Build history of the part. All positions in model axes, mm. Face numbers are marked on the shaded views. A direction names the side the tool comes from. Round coordinates to 2 decimals unless told otherwise and drop trailing zeros. Order: outer loops, then holes, each group sorted by start corner. A loop starts at its lowest first (then second) coordinate and runs counter-clockwise, first axis right, second up. Notation, with made-up numbers: M 8.5,-0.5 L 39.5,-0.5 A21 cw 39.5,7.5 Z; hole C 12.5,46 d6. An arc over 180 degrees is marked long. One line per item, written item: value. Start each with the question number.
Item 1: Two-plate mould, pull along Y, no slides. Class the marked faces 3, 4, 5 and 6: +Y half, -Y half, draft (parallel to the pull), parting line (faces both ways), or undercut.
Item 2: Band-saw the part on A-A, the plane x = 0. Write the cut outline in (y, z).
Item 3: Band-saw the part on C-C, the plane y = -4. Write the cut outline in (x, z), then the cut area to 3 significant figures.
Item 4: Probe L1, parallel to Y at x = 0, z = 0.4; L2, parallel to X at y = -4, z = 0.7; L3, parallel to Z at x = -2, y = -5.25. List the from-to ranges inside material, lowest first.
Item 5: Band-saw the part on D-D, the plane z = 1.75. Write the cut outline in (x, y).
Item 6: Pin check, flat tips, straight feed: pin 1 (4 mm diameter, centred on x = 6.5, y = -4, fed in from +Z); pin 2 (4 mm diameter, centred on x = 2, z = 6.5, fed in from -Y); pin 3 (2 mm diameter, centred on x = 0.5, y = -6, fed in from +Z). Stop position of each tip, or through.
Item 7: Tool access for the marked faces 1 and 2: list every direction of +Z, -Z, +X, -X, +Y, -Y with a clear straight run to the whole face (end or side of a thin tool).
Item 8: Band-saw the part on B-B, the plane y = 8. Write the cut outline in (x, z).
```python
from build123d import *

# Parameters (mm, degrees)
SKETCH_1_R               = 3
SKETCH_1_R_2             = 1.65
EXTRUDE_1_DEPTH          = 4
CUT_EXTRUDE_2_DEPTH      = 6.830951895
PATTERN_CIRCULAR_1_COUNT = 9
SKETCH_2_R               = 5
EXTRUDE_2_DEPTH          = 4
SKETCH_3_R               = 12.5
SKETCH_3_R_2             = 1.8
SKETCH_3_R_3             = 5
EXTRUDE_4_DEPTH          = 4
CUT_EXTRUDE_START        = 4
SKETCH_3_3_R             = 2.5
CUT_EXTRUDE_3_DEPTH      = 3
SKETCH_4_R               = 1.4
EXTRUDE_5_DEPTH          = 12.5


with BuildPart() as part:
    # 草图1 → 凸台-拉伸1 (new body)
    with BuildSketch(Plane.XY):
        Circle(SKETCH_1_R)
        Circle(SKETCH_1_R_2, mode=Mode.SUBTRACT)
    extrude(amount=EXTRUDE_1_DEPTH)

    # 草图1<3> → 切除-拉伸2 (cut, through all)
    with BuildSketch(Plane.XY):
        with BuildLine():
            Line((1.583201231, 0.595370355), (1.54440693, 0.580781573))
            ThreePointArc((1.54440693, 0.580781573), (1.623387112, 0.295151288), (1.65, 0))
            ThreePointArc((1.65, 0), (1.623387112, -0.295151288), (1.54440693, -0.580781573))
            Line((1.54440693, -0.580781573), (1.583201231, -0.595370355))
            add(Edge.make_bspline(
                [(1.583201231, -0.595370355), (1.595268082, -0.599908151), (1.629927649, -0.609960022), (1.698544644, -0.618780808), (1.810680065, -0.617601716), (1.954246735, -0.59352555), (2.132298369, -0.536822163), (2.302941373, -0.452472776), (2.42578745, -0.372108406), (2.505673341, -0.310927028), (2.533645284, -0.288342805)],
                knots=[0, 0, 0, 0, 0, 0.005604068, 0.015718248, 0.029959916, 0.048733667, 0.068727063, 0.096888892, 0.112551479, 0.112551479, 0.112551479, 0.112551479, 0.112551479], degree=4))
            ThreePointArc((2.533645284, -0.288342805), (2.545908038, -0.144403125), (2.55, 0))
            ThreePointArc((2.55, 0), (2.545908038, 0.144403125), (2.533645284, 0.288342805))
            add(Edge.make_bspline(
                [(1.583201231, 0.595370355), (1.595268082, 0.599908151), (1.629927649, 0.609960022), (1.698544644, 0.618780808), (1.810680065, 0.617601716), (1.954246735, 0.59352555), (2.132298369, 0.536822163), (2.302941373, 0.452472776), (2.42578745, 0.372108406), (2.505673341, 0.310927028), (2.533645284, 0.288342805)],
                knots=[0, 0, 0, 0, 0, 0.005604068, 0.015718248, 0.029959916, 0.048733667, 0.068727063, 0.096888892, 0.112551479, 0.112551479, 0.112551479, 0.112551479, 0.112551479], degree=4))
        make_face()
    cut_extrude_2 = extrude(amount=CUT_EXTRUDE_2_DEPTH, mode=Mode.SUBTRACT)

    # 阵列(圆周)1: 切除-拉伸2 ×9 about axis
    pattern_circular_1_axis = Axis((0, 0, 4), (0, 0, 1))
    for i in range(1, PATTERN_CIRCULAR_1_COUNT):
        add(cut_extrude_2.rotate(pattern_circular_1_axis, i * 360 / PATTERN_CIRCULAR_1_COUNT), mode=Mode.SUBTRACT)

    # 草图2 → 凸台-拉伸2 (add)
    with BuildSketch(Plane(origin=(0, 0, 0), x_dir=(-1, 0, 0), z_dir=(0, 0, -1))):
        Circle(SKETCH_2_R)
    extrude(amount=-EXTRUDE_2_DEPTH)

    # 草图3 → 凸台-拉伸4 (add)
    with BuildSketch(Plane.XY):
        Circle(SKETCH_3_R)
        with Locations((0, 8)):
            Circle(SKETCH_3_R_2, mode=Mode.SUBTRACT)
        with Locations((6.92820323, -4)):
            Circle(SKETCH_3_R_2, mode=Mode.SUBTRACT)
        with Locations((-6.92820323, -4)):
            Circle(SKETCH_3_R_2, mode=Mode.SUBTRACT)
        Circle(SKETCH_3_R_3, mode=Mode.SUBTRACT)
    extrude(amount=EXTRUDE_4_DEPTH)

    # 草图3<3> → 切除-拉伸3 (cut)
    with BuildSketch(Plane.XY.offset(CUT_EXTRUDE_START)):
        with Locations((0, 8)):
            Circle(SKETCH_3_3_R)
        with Locations((6.92820323, -4)):
            Circle(SKETCH_3_3_R)
        with Locations((-6.92820323, -4)):
            Circle(SKETCH_3_3_R)
    extrude(amount=-CUT_EXTRUDE_3_DEPTH, mode=Mode.SUBTRACT)

    # 草图4 → 凸台-拉伸5 (add)
    with BuildSketch(Plane.XY.offset(4)):
        Circle(SKETCH_4_R)
    extrude(amount=EXTRUDE_5_DEPTH)


solid = part.part
```
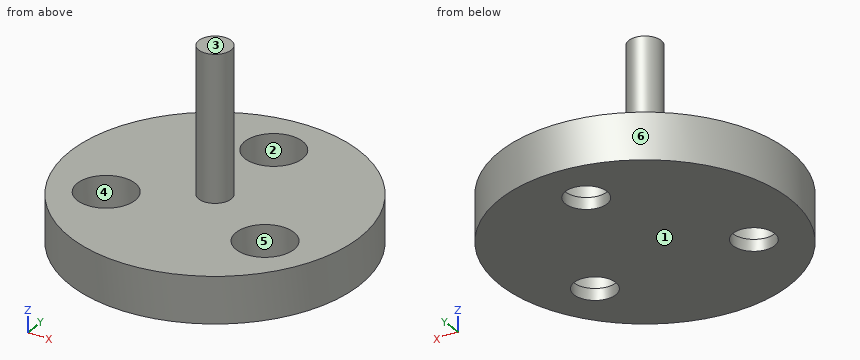
Output:
1. face 3: draft
1. face 4: undercut
1. face 5: undercut
1. face 6: parting line
2. outline: M -12.5,0 L 6.2,0 L 6.2,1 L 5.5,1 L 5.5,4 L 1.4,4 L 1.4,16.5 L -1.4,16.5 L -1.4,4 L -12.5,4 Z; M 9.8,0 L 12.5,0 L 12.5,4 L 10.5,4 L 10.5,1 L 9.8,1 Z
3. outline: M -11.84,0 L -8.73,0 L -8.73,1 L -9.43,1 L -9.43,4 L -11.84,4 Z; M -5.13,0 L 5.13,0 L 5.13,1 L 4.43,1 L 4.43,4 L -4.43,4 L -4.43,1 L -5.13,1 Z; M 8.73,0 L 11.84,0 L 11.84,4 L 9.43,4 L 9.43,1 L 8.73,1 Z
3. area: 57.5 mm²
4. L1: y = -12.5 to 6.2, 9.8 to 12.5
4. L2: x = -11.84 to -8.73, -5.13 to 5.13, 8.73 to 11.84
4. L3: z = 0 to 4
5. outline: C 0,0 d25; hole C -6.93,-4 d5; hole C 0,8 d5; hole C 6.93,-4 d5
6. pin 1: stops at z = 1
6. pin 2: stops at y = -1.4
6. pin 3: stops at z = 4
7. face 1: -Z, +X, -X, +Y, -Y
7. face 2: +Z
8. outline: M -9.6,0 L -1.8,0 L -1.8,1 L -2.5,1 L -2.5,4 L -9.6,4 Z; M 1.8,0 L 9.6,0 L 9.6,4 L 2.5,4 L 2.5,1 L 1.8,1 Z
